Model file for the job. Use its own axes, mm. Round coordinates to 2 decimals unless told otherwise and drop trailing zeros. Order: outer loops, then holes, each group sorted by start corner. A loop starts at its lowest first (then second) coordinate and runs counter-clockwise, first axis right, second up. Notation, with made-up numbers: (80.5, -3.75) -> (112.5, -3.75) arc R29 cw to (112.5, 28.25) -> close; hole circle Ø8 at (-2.5, 68). An arc over 180 degrees is marked (long way). Put each result on its own line as item: value. Start each with the question number.
Q1. Cut at A-A, the plane y = 2.3. List the corners of the cut face in (x, z).
Q2. Cut at C-C, the plane z = 356. List the corners of the cut face in (x, y).
Q3. Flat gauge pins, fed straight in: P1, Ø1, axis at y = 1.5, z = 120, coming from the +X side; P2, Ø1.2, axis at y = 1.5, z = 18, coming from the -X side; P3, Ø1, axis at x = -135, y = 3, coming from the +Z side. Where does each tip first touch, or does it go through?
Q4. Probe L1, parallel to X at y = 2.8, z = 28.5; L2, parallel to X at y = 2.1, z = 222.5; L3, parallel to X at y = 2.75, z = 64. List the from-to ranges inside material, lowest first.
Q5. Cut at B-B, the plane x = -66. List the corners of the cut face in (y, z), and give its area (3 significant figures).
from build123d import *

# Parameters (mm, degrees)
BOSS_EXTRUDE1_DEPTH = 4
FILLET1_R           = 1


with BuildPart() as part:
    # Sketch1 → Boss-Extrude1 (new body)
    with BuildSketch(Plane(origin=(0, 0, 0), x_dir=(-1, 0, 0), z_dir=(0, 1, 0))):
        Polygon((0, 0), (280, 0), (362.098214286, 427.182494036), align=None)
        with BuildLine():
            Line((207.9, 32.9), (207.9, 7.1))
            ThreePointArc((207.9, 7.1), (210, 5), (212.1, 7.1))
            Line((212.1, 7.1), (212.1, 32.9))
            ThreePointArc((212.1, 32.9), (210, 35), (207.9, 32.9))
        make_face(mode=Mode.SUBTRACT)
        with BuildLine():
            Line((132.1, 32.9), (132.1, 7.1))
            ThreePointArc((132.1, 7.1), (130, 5), (127.9, 7.1))
            Line((127.9, 7.1), (127.9, 32.9))
            ThreePointArc((127.9, 32.9), (130, 35), (132.1, 32.9))
        make_face(mode=Mode.SUBTRACT)
        with BuildLine():
            Line((277.666908222, 151.054979007), (303.003249248, 146.185705608))
            ThreePointArc((303.003249248, 146.185705608), (305.46184577, 147.851629717), (303.795921661, 150.31022624))
            Line((303.795921661, 150.31022624), (278.459580636, 155.179499639))
            ThreePointArc((278.459580636, 155.179499639), (276.000984113, 153.51357553), (277.666908222, 151.054979007))
        make_face(mode=Mode.SUBTRACT)
        with BuildLine():
            Line((289.783472261, 214.101222954), (315.119813287, 209.231949555))
            ThreePointArc((315.119813287, 209.231949555), (316.785737396, 206.773353032), (314.327140873, 205.107428923))
            Line((314.327140873, 205.107428923), (288.990799848, 209.976702322))
            ThreePointArc((288.990799848, 209.976702322), (287.324875738, 212.435298845), (289.783472261, 214.101222954))
        make_face(mode=Mode.SUBTRACT)
    extrude(amount=BOSS_EXTRUDE1_DEPTH)

    # Fillet1
    fillet1_edges = [part.edges().sort_by_distance(p)[0] for p in [
        (-362.098214286, 2, 427.182494036),
        (-280, 2, 0),
        (0, 2, 0),
    ]]
    fillet(fillet1_edges, radius=FILLET1_R)


solid = part.part
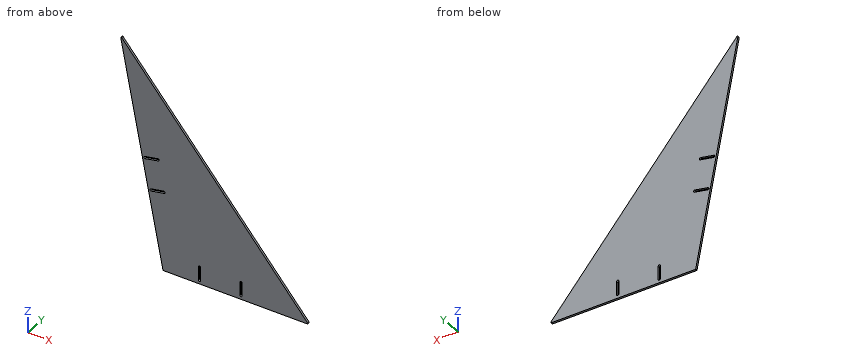
Ans:
1. outline: (-361.38, 423.44) -> (-280.16, 0.81) arc R1 ccw to (-279.17, 0) -> (-2.16, 0) arc R1 ccw to (-1.4, 1.65) -> (-359.63, 424.28) arc R1 ccw to start; hole (-315.12, 209.23) arc R2.1 ccw to (-314.33, 205.11) -> (-288.99, 209.98) arc R2.1 ccw to (-289.78, 214.1) -> close; hole (-303.8, 150.31) arc R2.1 ccw to (-303, 146.19) -> (-277.67, 151.05) arc R2.1 ccw to (-278.46, 155.18) -> close; hole (-212.1, 7.1) arc R2.1 ccw to (-207.9, 7.1) -> (-207.9, 32.9) arc R2.1 ccw to (-212.1, 32.9) -> close; hole (-132.1, 7.1) arc R2.1 ccw to (-127.9, 7.1) -> (-127.9, 32.9) arc R2.1 ccw to (-132.1, 32.9) -> close
2. outline: (-348.42, 0) -> (-301.76, 0) -> (-301.76, 4) -> (-348.42, 4) -> close
3. P1: stops at x = -101.29
3. P2: stops at x = -283.57
3. P3: stops at z = 159.86
4. L1: x = -285.48 to -212.1, -207.9 to -132.1, -127.9 to -24.16
4. L2: x = -322.76 to -188.6
4. L3: x = -292.3 to -54.25
5. outline: (0, 0) -> (4, 0) -> (4, 77.86) -> (0, 77.86) -> close
5. area: 311 mm^2
